Check sheet for the modelled part. Datum: model origin and axes. Units: mm. Round coordinates to 2 decimals unless told otherwise and drop trailing zeros. Loops run counter-clockwise (first coordinate to the right, second up) from the corner with the lowest first, then second, coordinate; pieces in that order, holes last. Notation, with made-up numbers: (1, 8) -> (33, 8) arc R25 ccw to (33, 30) -> close; hole circle Ø10 at (28.5, -5). An arc over 180 degrees is marked (long way). One line per question, with ' | ' between items.
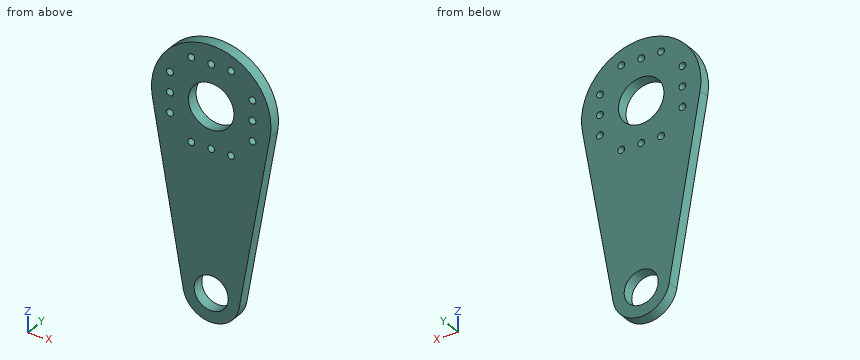
```python
from build123d import *

# Parameters (mm, degrees)
CROQUIS1_R              = 4
CROQUIS1_R_2            = 3
SALIENTE_EXTRUIR1_DEPTH = 2
SKETCH1_R               = 0.6
CUT_EXTRUDE1_DEPTH      = 2
CIRPATTERN1_COUNT       = 4


with BuildPart() as part:
    # Croquis1 → Saliente-Extruir1 (new body)
    with BuildSketch(Plane(origin=(0, 0, 0), x_dir=(1, 0, 0), z_dir=(0, 1, 0))):
        with BuildLine():
            Line((4.925593833, 32.859375), (10.34374705, 1.8046875))
            ThreePointArc((10.34374705, 1.8046875), (0, -10.5), (-10.34374705, 1.8046875))
            Line((-10.34374705, 1.8046875), (-4.925593833, 32.859375))
            ThreePointArc((-4.925593833, 32.859375), (0, 37), (4.925593833, 32.859375))
        make_face()
        Circle(CROQUIS1_R, mode=Mode.SUBTRACT)
        with Locations((0, 32)):
            Circle(CROQUIS1_R_2, mode=Mode.SUBTRACT)
    extrude(amount=SALIENTE_EXTRUIR1_DEPTH)

    # Sketch1 → Cut-Extrude1 (cut)
    with BuildSketch(Plane(origin=(0, 2, 0), x_dir=(1, 0, 0), z_dir=(0, 1, 0))):
        with Locations((0, 7.25)):
            Circle(SKETCH1_R)
        with Locations((-3.5, 7.25)):
            Circle(SKETCH1_R)
        with Locations((3.5, 7.25)):
            Circle(SKETCH1_R)
    cut_extrude1 = extrude(amount=-CUT_EXTRUDE1_DEPTH, mode=Mode.SUBTRACT)

    # CirPattern1: Cut-Extrude1 ×4 about axis
    cirpattern1_axis = Axis((0, 0, 0), (0, 1, 0))
    for i in range(1, CIRPATTERN1_COUNT):
        add(cut_extrude1.rotate(cirpattern1_axis, i * 360 / CIRPATTERN1_COUNT), mode=Mode.SUBTRACT)


solid = part.part
```
(1) Sectioned sample at A-A, the plane x = 0. Record the cut outline in (y, z).
Answer:
outline: (0, -37) -> (2, -37) -> (2, -35) -> (0, -35) -> close; (0, -29) -> (2, -29) -> (2, -7.85) -> (0, -7.85) -> close; (0, -6.65) -> (2, -6.65) -> (2, -4) -> (0, -4) -> close; (0, 4) -> (2, 4) -> (2, 6.65) -> (0, 6.65) -> close; (0, 7.85) -> (2, 7.85) -> (2, 10.5) -> (0, 10.5) -> close
(2) Sectioned sample at B-B, the plane z = -3.5. Record the cut outline in (x, y), and give its area (3 significant figures).
Answer:
outline: (-10.05, 0) -> (-7.85, 0) -> (-7.85, 2) -> (-10.05, 2) -> close; (-6.65, 0) -> (-1.94, 0) -> (-1.94, 2) -> (-6.65, 2) -> close; (1.94, 0) -> (6.65, 0) -> (6.65, 2) -> (1.94, 2) -> close; (7.85, 0) -> (10.05, 0) -> (10.05, 2) -> (7.85, 2) -> close | area: 27.6 mm2
(3) Sectioned sample at D-D, the plane x = 7.25. Record the cut outline in (y, z).
Answer:
outline: (0, -19.54) -> (2, -19.54) -> (2, -4.1) -> (0, -4.1) -> close; (0, -2.9) -> (2, -2.9) -> (2, -0.6) -> (0, -0.6) -> close; (0, 0.6) -> (2, 0.6) -> (2, 2.9) -> (0, 2.9) -> close; (0, 4.1) -> (2, 4.1) -> (2, 7.6) -> (0, 7.6) -> close
(4) Go/stop test with a flat-tipped pin: pin 1 (1.6 mm diameter, centred on x = 0, z = -7.25, fed in from +Y). Record where the tip stops, or that it passes through.
Answer:
pin 1: stops at y = 2
(5) Scan lines: probe 1 along Z at (x, y) = (0, 1.25); probe 2 along Z at (x, y) = (-2.25, 0.15); probe 3 along Z at (x, y) = (-1, 1.6). Record each from-to range of solid material in increasing order.
Answer:
probe 1: z = -37 to -35, -29 to -7.85, -6.65 to -4, 4 to 6.65, 7.85 to 10.5 | probe 2: z = -36.47 to -33.98, -30.02 to -3.31, 3.31 to 10.26 | probe 3: z = -36.9 to -34.83, -29.17 to -3.87, 3.87 to 10.45
(6) Sectioned sample at C-C, the plane y = 1.45. Count the separate pieces of the cut face and the enclosed holes in it, and give its area (3 significant figures).
Answer:
separate pieces: 1 | enclosed holes: 14 | area: 624 mm2
